Design review of the part shown in the three views and the two pictorial views. Dimensions are in mm from the part's minimum x, y and z. A direction names the side the tool comes from. Round coordinates to 2 decimals unless told otherwise and drop trailing zeros. Loops run counter-clockwise (first coordinate to the right, second up) from the corner with the lowest first, then second, coordinate; pieces in that order, holes last. Notation, with made-up numbers: (1, -19) - (38, -19) arc R18 cw to (38, -15) - close; hole circle Ø11 at (7, 19.25). An arc over 180 degrees is marked (long way). Return JSON: item names as keys, results as strings. Group by question number.
(1) We need section A-A, the plane z = 7. Give the number of separate pieces and of enclosed holes in the cut face, and give its area (3 significant figures).
(2) Wall thickness on L1, parallel to X at y = 1.55, z = 7; L2, parallel to Z at x = 5, y = 1.65; L3, parallel to X at y = 20, z = 10.75: over which ranges is each line inside the solid? List them lowest first. Write a range as [from, to].
(3) The part is to be moulded in two halves that separate along Z. For the marked faces 1, 2 and 3, say which applies: pulls with the +Z half, pulls with the -Z half, needs draft (parallel to the pull), parting line crosses it, or undercut.
(4) For the marked faces 4, 5 and 6, list the 3-axis set-ups (+Z, -Z, +X, -X, +Y, -Y) from which the entire face can be reached by the end or side of a thin tool; tool diameter is ignored.
(5) We need section B-B, the plane y = 20. Write out the cut boundary in (x, z), and give its area (3 significant figures).
(6) Clearance check with flat-ended pins moving along their axes: pin 1 (4 mm diameter, centred on y = 18, z = 8.5, fed in from -X); pin 2 (6 mm diameter, centred on x = 5, z = 7, fed in from +Y); pin 3 (4 mm diameter, centred on y = 14, z = 6, fed in from +X); pin 4 (6 mm diameter, centred on x = 27.5, z = 3.5, fed in from -Y). State where each tip first meets the part, or that it passes through.
(7) We need section C-C, the plane x = 5. Write out the cut boundary in (y, z).
(8) We need section D-D, the plane z = 2. Write out the cut boundary in (x, y) (1 decimal).
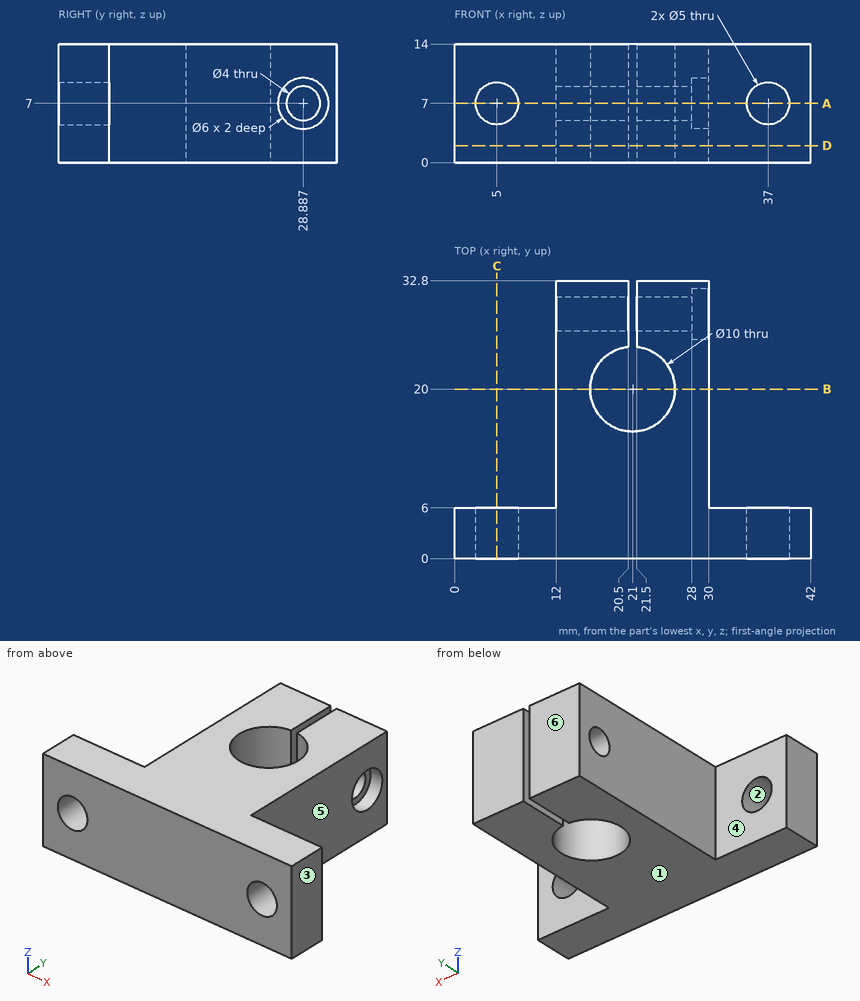
Solutions:
{
 "1": {"separate pieces": "5", "enclosed holes": "0", "area": "516 mm^2"},
 "2": {"L1": "[0, 2.5], [7.5, 34.5], [39.5, 42]", "L2": "[0, 4.5], [9.5, 14]", "L3": "[12, 16], [26, 30]"},
 "3": {"face 1": "pulls with the -Z half", "face 2": "undercut", "face 3": "needs draft"},
 "4": {"face 4": "+Z, -Z, -X, +Y", "face 5": "+Z, -Z, +X, +Y", "face 6": "+Z, -Z, +X, -X, +Y"},
 "5": {"outline": "(12, 0) - (16, 0) - (16, 14) - (12, 14) - close; (26, 0) - (30, 0) - (30, 14) - (26, 14) - close", "area": "112 mm^2"},
 "6": {"pin 1": "x = 12", "pin 2": "y = 6", "pin 3": "x = 30", "pin 4": "y = 0"},
 "7": {"outline": "(0, 0) - (6, 0) - (6, 4.5) - (0, 4.5) - close; (0, 9.5) - (6, 9.5) - (6, 14) - (0, 14) - close"},
 "8": {"outline": "(0, 0) - (42, 0) - (42, 6) - (30, 6) - (30, 32.8) - (21.5, 32.8) - (21.5, 25) arc R5 cw (long way) to (20.5, 25) - (20.5, 32.8) - (12, 32.8) - (12, 6) - (0, 6) - close"}
}
